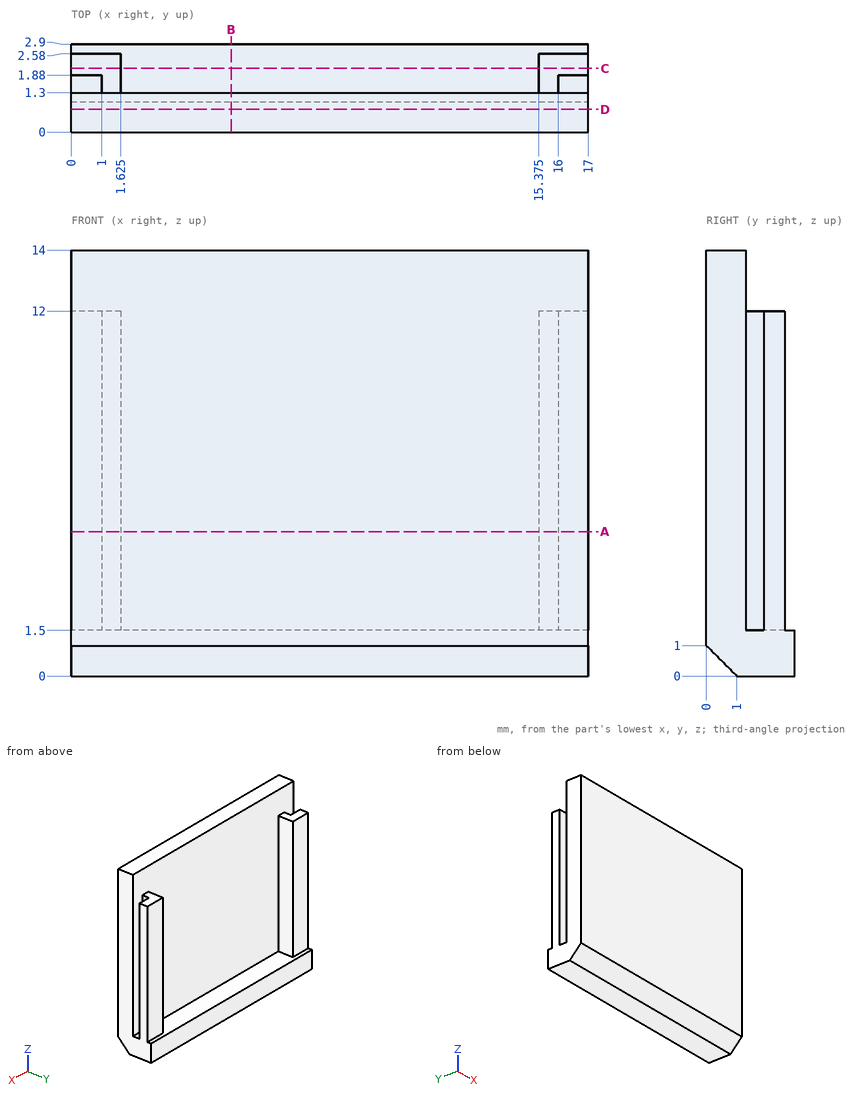
Could you check a few things on this drawing? It's one solid part, dimensions in mm from its lowest x, y, z. Coordinates: 2 decimals unless noted, no trailing zeros. Order: outer loops, then holes, each group sorted by start corner. A loop starts at its lowest first (then second) coordinate and runs counter-clockwise, first axis right, second up.
1. I'm going to push flat-ended pins straight in: pin 1 (0.5 mm diameter, centred on x = 5.5, y = 2.5, fed in from +Z); pin 2 (1.8 mm diameter, centred on x = 1, z = 6, fed in from +Y); pin 3 (2 mm diameter, centred on x = 3, z = 8.5, fed in from +Y). Where does each tip first touch, or does it pass through?
2. If we section it at D-D (y = 0.75): Please give me the cut outline in (x, z).
3. If we section it at A-A (z = 4.75): Please give me the cut outline in (x, y) (3 decimals), then the cut area to 3 significant figures.
4. If we section it at B-B (x = 5.25): Please give me the cut outline in (y, z), then the cut area to 3 significant figures.
5. I need wall thicknesses on line 1 (X direction, y = 2, z = 10.25) (3 decimals); line 2 (X direction, y = 1.7, z = 6.5) (3 decimals); line 3 (Z direction, x = 15.75, y = 1.45). Which ranges of each line are inside material? Lowest first, please.
6. If we section it at C-C (y = 2.1): Please give me the cut outline in (x, z) (3 decimals).
Entries:
1. pin 1: stops at z = 1.5
1. pin 2: stops at y = 2.58
1. pin 3: stops at y = 1.3
2. outline: (0, 0.25) - (17, 0.25) - (17, 14) - (0, 14) - close
3. outline: (0, 0) - (17, 0) - (17, 1.3) - (16, 1.3) - (16, 1.88) - (17, 1.88) - (17, 2.58) - (15.375, 2.58) - (15.375, 1.3) - (1.625, 1.3) - (1.625, 2.58) - (0, 2.58) - (0, 1.88) - (1, 1.88) - (1, 1.3) - (0, 1.3) - close
3. area: 25.1 mm2
4. outline: (0, 1) - (1, 0) - (2.9, 0) - (2.9, 1.5) - (1.3, 1.5) - (1.3, 14) - (0, 14) - close
4. area: 20.1 mm2
5. line 1: x = 0 to 1.625, 15.375 to 17
5. line 2: x = 1 to 1.625, 15.375 to 16
5. line 3: z = 0 to 12
6. outline: (0, 0) - (17, 0) - (17, 12) - (15.375, 12) - (15.375, 1.5) - (1.625, 1.5) - (1.625, 12) - (0, 12) - close
